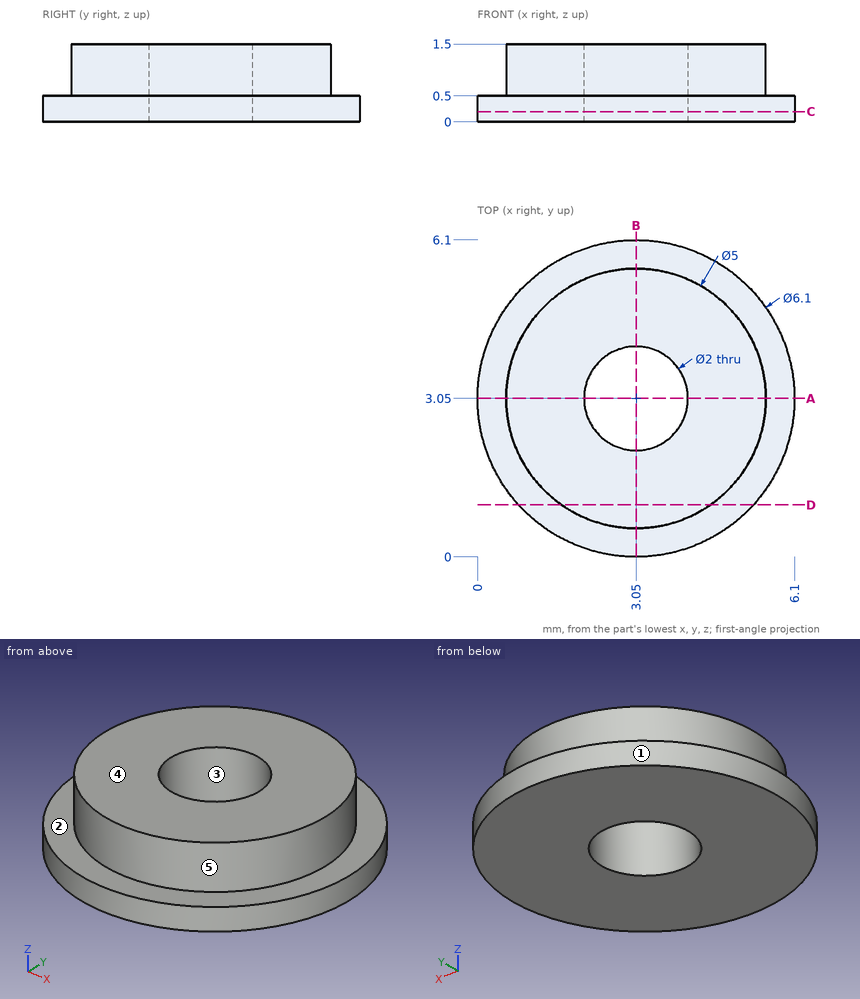
For this review, use the dimensioned drawing (mm, ordinates from the lowest corner) and the shaded views. A direction names the side the tool comes from. Round coordinates to 2 decimals unless told otherwise and drop trailing zeros. Order: outer loops, then holes, each group sorted by start corner. A loop starts at its lowest first (then second) coordinate and runs counter-clockwise, first axis right, second up. Notation, with made-up numbers: M 20,52 L 75,52 A4 ccw 75,59 Z; hole C -8.75,-36.75 d7. An arc over 180 degrees is marked long. Write each question's results on one line, items separated by ' | '. Start each with the question number.
1. Add section D-D (y = 1). State the section outline as (x, z) points, then the cut area to 3 significant figures.
2. Tool access review of the marked faces 4 and 5: name each direction out of +Z, -Z, +X, -X, +Y, -Y from which nothing blocks a thin tool from reaching the whole face with its end or side.
3. Add section A-A (y = 3.05). State the section outline as (x, z) points, then the cut area to 3 significant figures.
4. Add section C-C (z = 0.2). State the section outline as (x, y) points.
5. Draft analysis for pull direction X (two halves, no side actions). For the marked faces 1, 2 and 3, state which applies: pulls with the +X half, pulls with the -X half, needs draft (parallel to the pull), parting line crosses it, or undercut.
6. To check wall thickness, follow L1, parallel to Y at x = 3.05, z = 0.8; L2, parallel to Y at x = 3.05, z = 0.45; L3, parallel to X at y = 2.5, z = 0.45. State the ranges of each line that lie inside material, in increasing order. Write a range as [from, to].
7. Clearance check with a flat-ended pin moving along its axis: pin 1 Ø1.6 at (x, y) = (3.05, 3.05) entering from +Z. State where the tip first meets the part, or that it passes through.
Output values:
1) outline: M 0.79,0 L 5.31,0 L 5.31,0.5 L 4.48,0.5 L 4.48,1.5 L 1.62,1.5 L 1.62,0.5 L 0.79,0.5 Z | area: 5.12 mm^2
2) face 4: +Z, +X, -X, +Y, -Y | face 5: +Z
3) outline: M 0,0 L 2.05,0 L 2.05,1.5 L 0.55,1.5 L 0.55,0.5 L 0,0.5 Z; M 4.05,0 L 6.1,0 L 6.1,0.5 L 5.55,0.5 L 5.55,1.5 L 4.05,1.5 Z | area: 5.05 mm^2
4) outline: C 3.05,3.05 d6.1; hole C 3.05,3.05 d2
5) face 1: parting line crosses it | face 2: needs draft | face 3: undercut
6) L1: [0.55, 2.05], [4.05, 5.55] | L2: [0, 2.05], [4.05, 6.1] | L3: [0.05, 2.21], [3.89, 6.05]
7) pin 1: through
